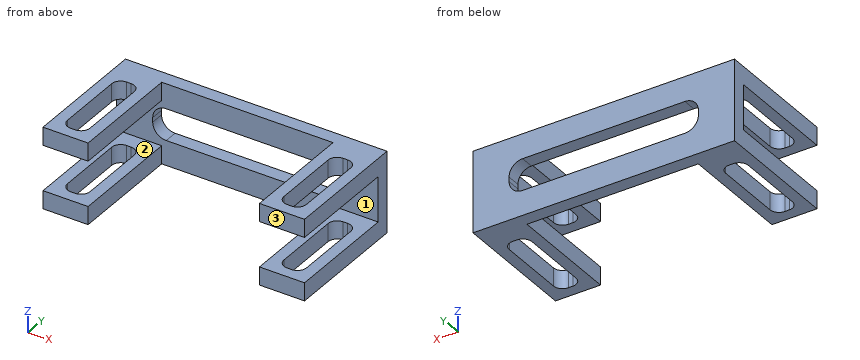
from build123d import *

# Parameters (mm, degrees)
F0_W     = 58
F0_H     = 18
F1_DEPTH = 3
F2_W     = 10
F2_H     = 4
F3_DEPTH = 25
F5_DEPTH = 3.001
F7_DEPTH = 18.001


with BuildPart() as f1:
    # F0 (on Front) → F1 (new body)
    with BuildSketch(Plane.XZ):
        with Locations((29, 9)):
            Rectangle(F0_W, F0_H)
    extrude(amount=F1_DEPTH)

    # F2 (on face) → F3 (join)
    with BuildSketch(Plane.XZ.offset(3)):
        with Locations((53, 16)):
            Rectangle(F2_W, F2_H)
        with Locations((53, 2)):
            Rectangle(F2_W, F2_H)
        with Locations((5, 2)):
            Rectangle(F2_W, F2_H)
        with Locations((5, 16)):
            Rectangle(F2_W, F2_H)
    extrude(amount=F3_DEPTH)

    # F4 (on face) → F5 (cut, through all)
    with BuildSketch(Plane.XZ.offset(3)):
        with BuildLine():
            Line((47, 12.5), (11, 12.5))
            ThreePointArc((11, 12.5), (8.87868, 11.62132), (8, 9.5))
            Line((8, 9.5), (8, 8.5))
            ThreePointArc((8, 8.5), (8.87868, 6.37868), (11, 5.5))
            Line((11, 5.5), (47, 5.5))
            ThreePointArc((47, 5.5), (49.12132, 6.37868), (50, 8.5))
            Line((50, 8.5), (50, 9.5))
            ThreePointArc((50, 9.5), (49.12132, 11.62132), (47, 12.5))
        make_face()
    extrude(amount=-F5_DEPTH, mode=Mode.SUBTRACT)

    # F6 (on face) → F7 (cut, through all)
    with BuildSketch(Plane.XY.offset(18)):
        with BuildLine():
            Line((5.5, -6.5), (4.5, -6.5))
            ThreePointArc((4.5, -6.5), (3.085786, -7.085786), (2.5, -8.5))
            Line((2.5, -8.5), (2.5, -23.5))
            ThreePointArc((2.5, -23.5), (3.085786, -24.914214), (4.5, -25.5))
            Line((4.5, -25.5), (5.5, -25.5))
            ThreePointArc((5.5, -25.5), (6.914214, -24.914214), (7.5, -23.5))
            Line((7.5, -23.5), (7.5, -8.5))
            ThreePointArc((7.5, -8.5), (6.914214, -7.085786), (5.5, -6.5))
        make_face()
        with BuildLine():
            Line((53.5, -6.5), (52.5, -6.5))
            ThreePointArc((52.5, -6.5), (51.085786, -7.085786), (50.5, -8.5))
            Line((50.5, -8.5), (50.5, -23.5))
            ThreePointArc((50.5, -23.5), (51.085786, -24.914214), (52.5, -25.5))
            Line((52.5, -25.5), (53.5, -25.5))
            ThreePointArc((53.5, -25.5), (54.914214, -24.914214), (55.5, -23.5))
            Line((55.5, -23.5), (55.5, -8.5))
            ThreePointArc((55.5, -8.5), (54.914214, -7.085786), (53.5, -6.5))
        make_face()
    extrude(amount=-F7_DEPTH, mode=Mode.SUBTRACT)


solid = f1.part
Can you work these out from the model? Positions are in its coordinate system, mm. Face numbers are marked on the shaded views. A direction names the side the tool comes from. Give positions to 0.01 mm unless a question says otherwise; leave off trailing zeros. Loops run counter-clockwise (first coordinate to the right, second up) from the corner with the lowest first, then second, coordinate; pieces in that order, holes last. Notation, with made-up numbers: M 18,-36 L 75,-36 A18 ccw 75,-17 Z; hole C 63.5,12 d10. An arc over 180 degrees is marked long. One line per item, written item: value. Start each with the question number.
1) If we section it at D-D, the plane z = 11.75: Write out the boundary of the cut face in (x, y).
2) If we section it at C-C, the plane z = 16.5: Write out the boundary of the cut face in (x, y), and give its area (3 significant figures).
3) If we section it at A-A, the plane y = -16.25: Give the number of separate pieces and of enclosed holes in the cut face, and give its area (3 significant figures).
4) I'm going to push flat-ended pins straight in: pin 1 (3 mm diameter, centred on x = 34, z = 15, fed in from -Y); pin 2 (2 mm diameter, centred on x = 46.5, y = -16, fed in from -Z). Where does each tip first touch, or does it pass through?
5) On a 3-axis mill with a long thin cutter (end or side, diameter ignored), from which of +Z, -Z, +X, -X, +Y, -Y can I reach the whole of each face in a straight line? I mean the marked faces 1, 2 and 3. Say none if no direction works.
6) If I drill on line 1 (X direction, y = -17, z = 15.5); line 2 (Z direction, x = 5, y = -6); line 3 (Y direction, x = 36, z = 4.75), over which ranges is the centre line in solid material (lowest first)? Write a range as [from, to].
7) If we section it at B-B, the plane x = 35.5: Write out the boundary of the cut face in (y, z).
Completed:
1. outline: M 0,-3 L 9.02,-3 L 9.02,0 L 0,0 Z; M 48.98,-3 L 58,-3 L 58,0 L 48.98,0 Z
2. outline: M 0,-28 L 10,-28 L 10,-3 L 48,-3 L 48,-28 L 58,-28 L 58,0 L 0,0 Z; hole M 2.5,-23.5 A2 ccw 4.5,-25.5 L 5.5,-25.5 A2 ccw 7.5,-23.5 L 7.5,-8.5 A2 ccw 5.5,-6.5 L 4.5,-6.5 A2 ccw 2.5,-8.5 Z; hole M 50.5,-23.5 A2 ccw 52.5,-25.5 L 53.5,-25.5 A2 ccw 55.5,-23.5 L 55.5,-8.5 A2 ccw 53.5,-6.5 L 52.5,-6.5 A2 ccw 50.5,-8.5 Z
2. area: 491 mm^2
3. separate pieces: 8
3. enclosed holes: 0
3. area: 80.0 mm^2
4. pin 1: stops at y = -3
4. pin 2: passes through
5. face 1: -Y
5. face 2: +X, -X, -Y
5. face 3: +Z, -Z, +X, -X, -Y
6. line 1: x = [0, 2.5], [7.5, 10], [48, 50.5], [55.5, 58]
6. line 2: z = [0, 4], [14, 18]
6. line 3: y = [-3, 0]
7. outline: M -3,0 L 0,0 L 0,5.5 L -3,5.5 Z; M -3,12.5 L 0,12.5 L 0,18 L -3,18 Z
